Drawing for the job (mm, zero at the part's lowest x, y, z). A direction names the side the tool comes from. Give positions to 0.01 mm unless a question says otherwise; leave off trailing zeros. Order: outer loops, then holes, each group sorted by start corner. A loop starts at its lowest first (then second) coordinate and runs counter-clockwise, first axis right, second up. Notation, with made-up numbers: (34.25, 55.25) - (77.25, 55.25) arc R20 cw to (77.25, 60.25) - close; hole circle Ø6 at (15, 32). An arc over 180 degrees is marked (long way). Use CSV: the item, a comma, the result in double quotes. Start each with the question number.
(1) Band-saw the part on C-C, the plane z = 69. Give the cut face in (x, y).
(2) Band-saw the part on B-B, the plane x = 21. Give the cut face in (y, z), then the cut area to 3 significant figures.
(3) Band-saw the part on A-A, the plane y = 9.25. Give the cut face in (x, z).
(4) Probe L1, parallel to X at y = 7, z = 40; L2, parallel to Y at x = 43, z = 22. List the from-to ranges inside material, lowest first.
(5) Pull direction Z, two halves, no side cores. Call the marked faces 1, 2 and 3: +Z half, -Z half, draft (parallel to the pull), parting line (faces both ways), or undercut.
(6) Tool access for the marked faces 4 and 5: list every direction of +Z, -Z, +X, -X, +Y, -Y with a clear straight run to the whole face (end or side of a thin tool).
(7) Band-saw the part on D-D, the plane x = 46.5. Give the cut face in (y, z), then the cut area to 3 significant figures.
(8) Drop a flat-ended pin along its axis: pin 1 Ø3 at (x, z) = (68, 29.5) entering from +Y. Give the stop position or say it passes through.
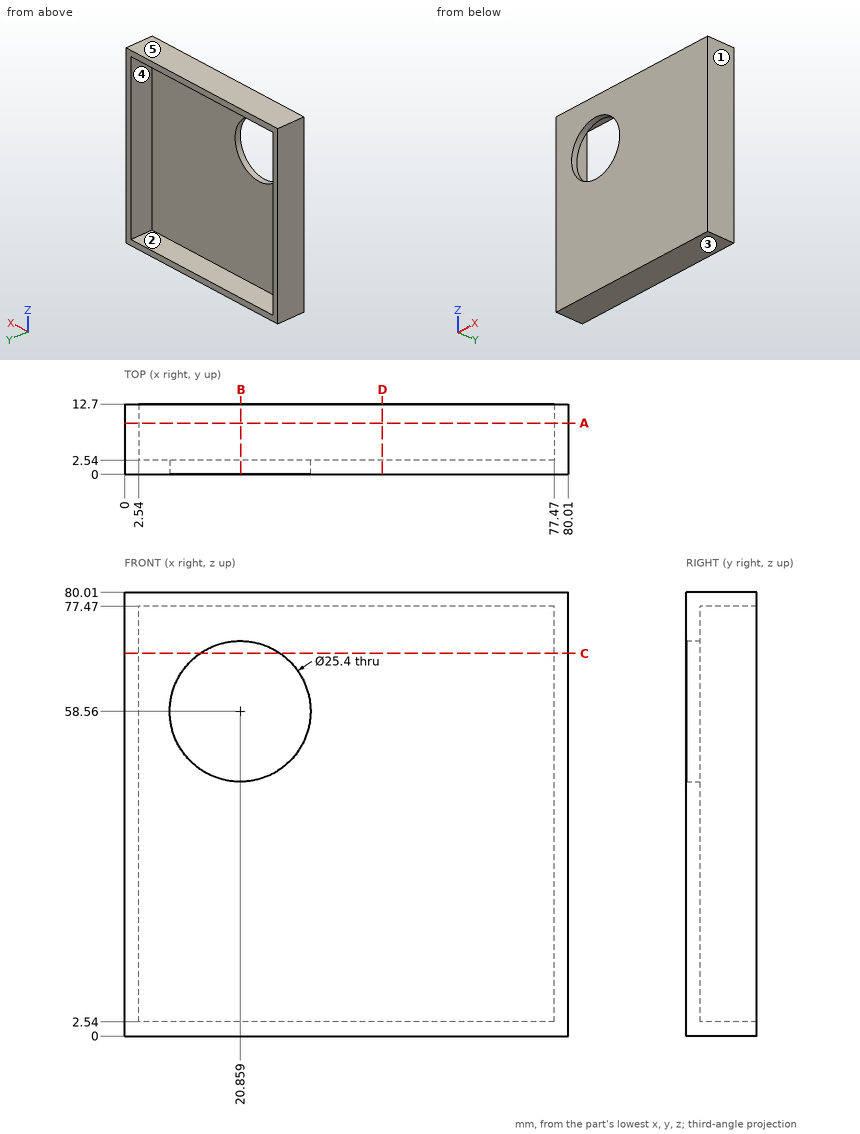
Answer block:
1,outline,"(0, 0) - (13.63, 0) - (13.63, 2.54) - (2.54, 2.54) - (2.54, 12.7) - (0, 12.7) - close; (28.09, 0) - (80.01, 0) - (80.01, 12.7) - (77.47, 12.7) - (77.47, 2.54) - (28.09, 2.54) - close"
2,outline,"(0, 0) - (12.7, 0) - (12.7, 2.54) - (2.54, 2.54) - (2.54, 45.86) - (0, 45.86) - close; (0, 71.26) - (2.54, 71.26) - (2.54, 77.47) - (12.7, 77.47) - (12.7, 80.01) - (0, 80.01) - close"
2,area,"190 mm2"
3,outline,"(0, 0) - (80.01, 0) - (80.01, 80.01) - (0, 80.01) - close; hole (2.54, 2.54) - (77.47, 2.54) - (77.47, 77.47) - (2.54, 77.47) - close"
4,L1,"x = 0 to 2.54, 77.47 to 80.01"
4,L2,"y = 0 to 2.54"
5,face 1,"draft"
5,face 2,"undercut"
5,face 3,"-Z half"
6,face 4,"+Y"
6,face 5,"+Z, +X, -X, +Y, -Y"
7,outline,"(0, 0) - (12.7, 0) - (12.7, 2.54) - (2.54, 2.54) - (2.54, 77.47) - (12.7, 77.47) - (12.7, 80.01) - (0, 80.01) - close"
7,area,"255 mm2"
8,pin 1,"stops at y = 2.54"
